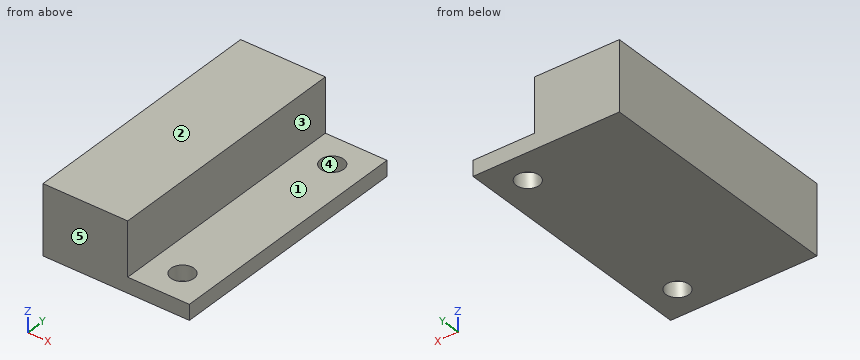
```python
from build123d import *

# Parameters (mm, degrees)
SKETCH1_W                 = 19
SKETCH1_H                 = 33
BOSS_EXTRUDE1_DEPTH       = 9
SKETCH3_W                 = 8
SKETCH3_H                 = 33
CUT_EXTRUDE1_DEPTH        = 7
F_3_0MM_DOWEL_HOLE1_D     = 3
F_3_0MM_DOWEL_HOLE1_DEPTH = 2


with BuildPart() as part:
    # Sketch1 → Boss-Extrude1 (new body)
    with BuildSketch(Plane.XY):
        with Locations((9.5, 16.5)):
            Rectangle(SKETCH1_W, SKETCH1_H)
    extrude(amount=BOSS_EXTRUDE1_DEPTH)

    # Sketch3 → Cut-Extrude1 (cut)
    with BuildSketch(Plane.XY.offset(9)):
        with Locations((15, 16.5)):
            Rectangle(SKETCH3_W, SKETCH3_H)
    extrude(amount=-CUT_EXTRUDE1_DEPTH, mode=Mode.SUBTRACT)

    # Ø3.0mm Dowel Hole1
    with Locations(Plane.XY.offset(2)):
        with Locations((15, 4), (15, 29)):
            Hole(F_3_0MM_DOWEL_HOLE1_D / 2, depth=F_3_0MM_DOWEL_HOLE1_DEPTH)


solid = part.part
```
Check sheet for the modelled part. Datum: model origin and axes. Units: mm. Face numbers are marked on the shaded views. A direction names the side the tool comes from. Round coordinates to 2 decimals unless told otherwise and drop trailing zeros. Loops run counter-clockwise (first coordinate to the right, second up) from the corner with the lowest first, then second, coordinate; pieces in that order, holes last. Notation, with made-up numbers: (-11, 41) - (13, 41) arc R34 cw to (13, 78) - close; hole circle Ø2 at (-34.75, 26). An arc over 180 degrees is marked (long way). Write item = value, one per line. Start each with the question number.
Q1. Section check D-D (z = 3). Record the boundary of the cut face in (x, y).
Q2. Thickness scan on L1, parallel to Y at x = 15, z = 1.3; L2, parallel to Z at x = 18, y = 4; L3, parallel to X at y = 22, z = 7.25. Record the ranges inside material, lowest first.
Q3. Section check A-A (x = 15). Record the boundary of the cut face in (y, z), plus the area to 3 significant figures.
Q4. Section check C-C (y = 12.5). Record the boundary of the cut face in (x, z), plus the area to 3 significant figures.
Q5. Release check for a two-part mould opening along Y. For the marked faces 3, 4 and 5 record: pulls with the +Y half, pulls with the -Y half, needs draft (parallel to the pull), parting line crosses it, or undercut.
Q6. Access from +Z, -Z, +X, -X, +Y, -Y to the whole of each face (thin tool, end or side, straight path). Record for the marked faces 1 and 2.
Q7. Depth check by flat-ended pin: P1, Ø2.5, axis at x = 13.5, y = 9.5, coming from the +Z side; P2, Ø3, axis at y = 27, z = 5, coming from the +X side; P3, Ø2.5, axis at x = 15, y = 29, coming from the +Z side. Enter the tip coordinate at first touch or a pass-through.
Q8. Section check B-B (y = 29). Record the boundary of the cut face in (x, z), plus the area to 3 significant figures.
Derived:
q1.outline = (0, 0) - (11, 0) - (11, 33) - (0, 33) - close
q2.L1 = 0 to 2.5, 5.5 to 27.5, 30.5 to 33
q2.L2 = 0 to 2
q2.L3 = 0 to 11
q3.outline = (0, 0) - (2.5, 0) - (2.5, 2) - (0, 2) - close; (5.5, 0) - (27.5, 0) - (27.5, 2) - (5.5, 2) - close; (30.5, 0) - (33, 0) - (33, 2) - (30.5, 2) - close
q3.area = 54.0 mm^2
q4.outline = (0, 0) - (19, 0) - (19, 2) - (11, 2) - (11, 9) - (0, 9) - close
q4.area = 115 mm^2
q5.face_3 = needs draft
q5.face_4 = undercut
q5.face_5 = pulls with the -Y half
q6.face_1 = +Z, +X, +Y, -Y
q6.face_2 = +Z, +X, -X, +Y, -Y
q7.P1 = 2
q7.P2 = 11
q7.P3 = through
q8.outline = (0, 0) - (13.5, 0) - (13.5, 2) - (11, 2) - (11, 9) - (0, 9) - close; (16.5, 0) - (19, 0) - (19, 2) - (16.5, 2) - close
q8.area = 109 mm^2
